Model file for the job. Use its own axes, mm. Face numbers are marked on the shaded views. A direction names the side the tool comes from. Give positions to 0.01 mm unless a question says otherwise; leave off trailing zeros. Loops run counter-clockwise (first coordinate to the right, second up) from the corner with the lowest first, then second, coordinate; pieces in that order, holes last. Notation, with made-up numbers: M 83,67.25 L 97,67.25 A25 ccw 97,96.25 Z; hole C -26,-3 d9. An arc over 180 degrees is marked long. Answer in a Markdown table with one row per item.
Autodesk Inventor part; units mm, degrees
ref_plane "Work Plane1" through (3.175, -7.0346, 3.175) normal (0, 1, 0) x (1, 0, 0)
ref_plane "YZ Plane" through (0, 0, 0) normal (1, 0, 0) x (0, 1, 0)
ref_plane "XZ Plane" through (0, 0, 0) normal (0, 1, 0) x (-1, 0, 0)
sketch "Sketch1" plane through (0, 0, 0) normal (0, 0, 1) x (1, 0, 0)
  line L0 (0, 12.0154) -> (19.05, 12.0154)
  line L1 (19.05, 12.0154) -> (19.05, -26.0846)
  line L2 (19.05, -26.0846) -> (0, -26.0846)
  line L3 (0, -26.0846) -> (0, 12.0154)
  circle A0 centre (9.525, 2.4904) radius 3.175
  circle A1 centre (9.525, -16.5596) radius 3.175
  point P0 (0, 0)
  dimension "d0" = 19.05
  dimension "d1" = 38.1
  dimension "d2" = 6.35
  dimension "d3" = 6.35
  dimension "d4" = 19.05
  dimension "d5" = 9.525
  dimension "d6" = 9.525
extrude "Extrusion1" add sketch "Sketch1" along normal blind 3.175
fillet "Fillet1" radius 3.175 2 edges at (0, 12.0154, 1.5875) (0, -26.0846, 1.5875)
sketch "Sketch2" plane through (19.05, 12.0154, 3.175) normal (0, 1, 0) x (1, 0, 0)
  circle A0 centre (0, -1.5875) radius 4.7625
  circle A1 centre (0, -1.5875) radius 4.7625
  line L0 (-15.875, 3.175) -> (0, 3.175)
  point P0 (-19.05, 3.175)
extrude "Extrusion2" add sketch "Sketch2" against normal blind 38.1
ref_plane "Work Plane1" through (3.175, -7.0346, 3.175) normal (0, 1, 0) x (1, 0, 0)
sketch "Sketch3" plane through (3.175, -7.0346, 3.175) normal (0, 1, 0) x (1, 0, 0)
  arc A0 (11.3849, 0) -> (15.875, 3.175) centre (15.875, -1.5875) ccw
  circle A1 centre (15.875, -1.5875) radius 4.7625
  point P0 (-3.175, 3.175)
extrude "Extrusion3" cut sketch "Sketch3" along normal mid plane 12.7
sketch "Sketch5" plane through (3.175, 12.0154, 3.175) normal (0, 1, 0) x (1, 0, 0)
  circle A0 centre (15.875, -1.5875) radius 2.3813
  point P0 (-3.175, 3.175)
  point P1 (15.875, -1.5875)
  dimension "d16" = 4.7625
extrude "Extrusion4" cut sketch "Sketch5" against normal blind 38.1
equation "\"d3\" = d2"
equation "\"d4\" = 0.5 * d1"
equation "\"d5\" = 0.25 * d1"
equation "\"d6\" = 0.5 * d0"
properties part number "hinge left" material "Brass, Soft Yellow"
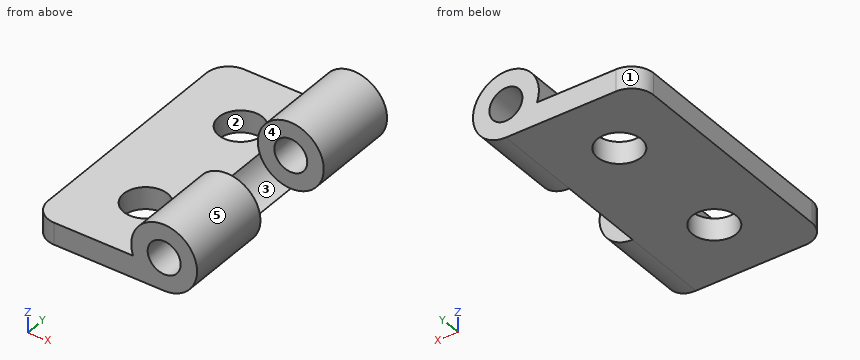
Q1. 3-axis set-ups, long thin cutter, end or side, ignore diameter. For the marked faces 4 and 5: which of +Z, -Z, +X, -X, +Y, -Y reach the whole face in a straight line?
Reported:
| item | result |
|---|---|
| face 4 | +Z, +X |
| face 5 | +Y, -Y |
Q2. Saw through at D-D (z = 6). Give the cut face in (x, y), and give its area (3 significant figures).
Reported:
| item | result |
|---|---|
| outline | M 14.45,-26.08 L 17.02,-26.08 L 17.02,-13.38 L 14.45,-13.38 Z; M 14.45,-0.68 L 17.02,-0.68 L 17.02,12.02 L 14.45,12.02 Z; M 21.08,-26.08 L 23.65,-26.08 L 23.65,-13.38 L 21.08,-13.38 Z; M 21.08,-0.68 L 23.65,-0.68 L 23.65,12.02 L 21.08,12.02 Z |
| area | 130 mm² |
Q3. Mould opens along X. For the marked faces 1, 2 and 3 say: released by +X, released by -X, zero draft, split by the parting line, or undercut.
Reported:
| item | result |
|---|---|
| face 1 | released by -X |
| face 2 | undercut |
| face 3 | released by +X |
Q4. Saw through at B-B (z = 2.75). Give the cut face in (x, y) (3 decimals).
Reported:
| item | result |
|---|---|
| outline | M 0,-22.91 A3.175 ccw 3.175,-26.085 L 17.777,-26.085 L 17.777,-13.385 L 14.734,-13.385 L 14.734,-0.685 L 17.777,-0.685 L 17.777,12.015 L 3.175,12.015 A3.175 ccw 0,8.84 Z; M 20.323,-26.085 L 23.366,-26.085 L 23.366,-13.385 L 20.323,-13.385 Z; M 20.323,-0.685 L 23.366,-0.685 L 23.366,12.015 L 20.323,12.015 Z; hole C 9.525,-16.56 d6.35; hole C 9.525,2.49 d6.35 |
Q5. Drop flat-ended pins along their axis: pin 1 (5.5 mm diameter, centred on x = 9.52, y = 2.49, fed in from +Z); pin 2 (1 mm diameter, centred on x = 16.5, y = 4.5, fed in from +Z); pin 3 (7.5 mm diameter, centred on x = 10, y = -13, fed in from +Z) (3 decimals). Give the stop position or say it passes through.
Reported:
| item | result |
|---|---|
| pin 1 | through |
| pin 2 | z = 9.06 |
| pin 3 | z = 3.175 |
Q6. Saw through at C-C (x = 19.75). Give the cut face in (y, z), and give its area (3 significant figures).
Reported:
| item | result |
|---|---|
| outline | M -26.08,0.05 L -13.38,0.05 L -13.38,2.49 L -26.08,2.49 Z; M -26.08,7.04 L -13.38,7.04 L -13.38,9.47 L -26.08,9.47 Z; M -0.68,0.05 L 12.02,0.05 L 12.02,2.49 L -0.68,2.49 Z; M -0.68,7.04 L 12.02,7.04 L 12.02,9.47 L -0.68,9.47 Z |
| area | 124 mm² |
Q7. Saw through at A-A (y = 3). Give the number of separate pieces and of enclosed holes in the cut face, and give its area (3 significant figures).
Reported:
| item | result |
|---|---|
| separate pieces | 2 |
| enclosed holes | 1 |
| area | 83.6 mm² |
Q8. Probe probe 1 along Y at (x, z) = (15.5, 6.25); probe 2 along Z at (x, y) = (19.05, -22) (3 decimals); probe 3 along Z at (x, y) = (1.5, -22.5) (3 decimals). List the from-to ranges inside material, lowest first.
Reported:
| item | result |
|---|---|
| probe 1 | -26.08 to -13.38, -0.68 to 12.02 |
| probe 2 | 0 to 2.381, 7.144 to 9.525 |
| probe 3 | 0 to 3.175 |
